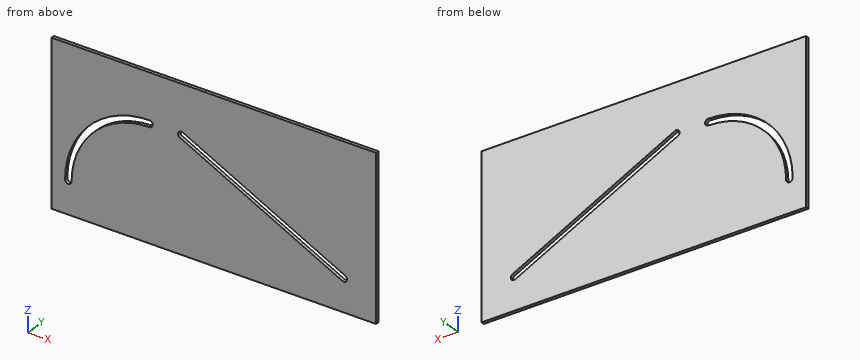
from build123d import *

# Parameters (mm, degrees)
ESQUISSE1_W             = 2000
ESQUISSE1_H             = 20
BOSS_EXTRU_1_DEPTH      = 1000
ENL_V_MAT_EXTRU_1_DEPTH = 2237.15741843


with BuildPart() as part:
    # Esquisse1 → Boss.-Extru.1 (new body)
    with BuildSketch(Plane.XY):
        with Locations((1000, 10)):
            Rectangle(ESQUISSE1_W, ESQUISSE1_H)
    extrude(amount=BOSS_EXTRU_1_DEPTH)

    # Esquisse2 → Enlèv. mat.-Extru.1 (cut, through all)
    with BuildSketch(Plane(origin=(0, 20, 0), x_dir=(1, 0, 0), z_dir=(0, 1, 0))):
        with BuildLine():
            Line((1808.94427191, -217.88854382), (808.94427191, -717.88854382))
            ThreePointArc((808.94427191, -717.88854382), (782.11145618, -708.94427191), (791.05572809, -682.11145618))
            Line((791.05572809, -682.11145618), (1791.05572809, -182.11145618))
            ThreePointArc((1791.05572809, -182.11145618), (1817.88854382, -191.05572809), (1808.94427191, -217.88854382))
        make_face()
        with BuildLine():
            ThreePointArc((83.245255668, -200), (235.549729451, -567.695526217), (603.245255668, -720))
            ThreePointArc((603.245255668, -720), (623.245255668, -700), (603.245255668, -680))
            ThreePointArc((603.245255668, -680), (263.834000698, -539.41125497), (123.245255668, -200))
            ThreePointArc((123.245255668, -200), (103.245255668, -180), (83.245255668, -200))
        make_face()
    extrude(amount=-ENL_V_MAT_EXTRU_1_DEPTH, mode=Mode.SUBTRACT)


solid = part.part
Part model, mm, in its own coordinate system. Coordinates: 2 decimals unless noted, no trailing zeros. Write each loop counter-clockwise with the first axis right and the second up, starting at its lowest first coordinate (ties: lowest second). Pieces come first, ordered by that corner, then holes. Notation, with made-up numbers: M 47.25,-19 L 74.25,-19 A24 cw 74.25,-3 Z; hole C -33.75,-12 d11. An arc over 180 degrees is marked long. Return JSON: item names as keys, results as strings.
1. Saw through at A-A, the plane z = 423. Write the cut outline in (x, y).
Determined:
{"outline": "M 0,0 L 133.49,0 L 133.49,20 L 0,20 Z; M 178.19,0 L 1309.28,0 L 1309.28,20 L 178.19,20 Z; M 1398.72,0 L 2000,0 L 2000,20 L 1398.72,20 Z"}
2. Probe L1, parallel to X at y = 12, z = 611.5; L2, parallel to X at y = 9.5, z = 210; L3, parallel to Z at x = 1411.5, y = 7.5. List the from-to ranges inside material, lowest first.
Determined:
{"L1": "0 to 285.33, 356.13 to 932.28, 1021.72 to 2000", "L2": "0 to 83.34, 123.35 to 1735.28, 1817.32 to 2000", "L3": "0 to 371.89, 416.61 to 1000"}
3. Saw through at B-B, the plane y = 7.75. Write the cut outline in (x, z).
Determined:
{"outline": "M 0,0 L 2000,0 L 2000,1000 L 0,1000 Z; hole M 83.25,200 A20 ccw 123.25,200 A480 cw 603.25,680 A20 ccw 603.25,720 A520 ccw Z; hole M 791.06,682.11 L 1791.06,182.11 A20 ccw 1808.94,217.89 L 808.94,717.89 A20 ccw Z"}
4. Saw through at C-C, the plane x = 1327.5. Write the cut outline in (y, z).
Determined:
{"outline": "M 0,0 L 20,0 L 20,413.89 L 0,413.89 Z; M 0,458.61 L 20,458.61 L 20,1000 L 0,1000 Z"}
